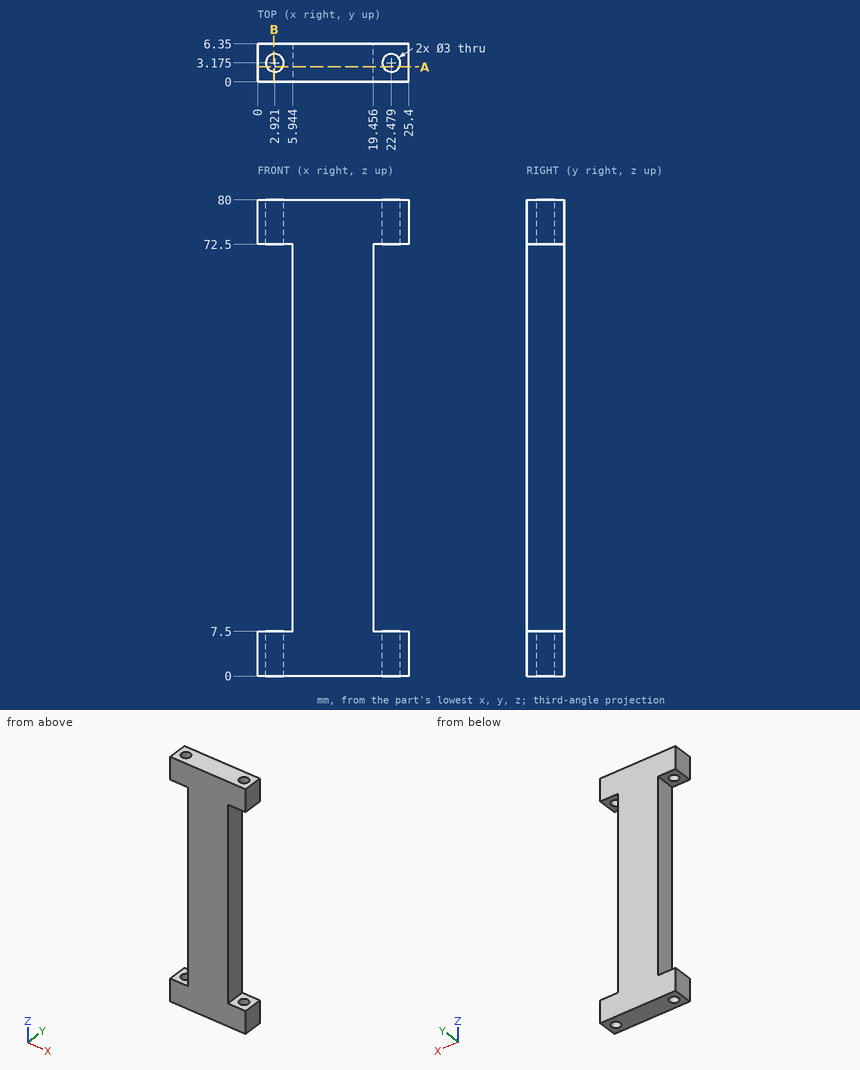
Here's the drawing with two shaded views (mm, measured from the low corner). I have some questions. Coordinates: 2 decimals unless noted, no trailing zeros. Loops run counter-clockwise (first coordinate to the right, second up) from the corner with the lowest first, then second, coordinate; pieces in that order, holes last. Notation, with made-up numbers: (65, 69) -> (79, 69) arc R18 ccw to (79, 86) -> close; hole circle Ø10 at (45.5, -36). An arc over 180 degrees is marked (long way). Answer in a Markdown table with one row per item.
(1) Imagine slicing it at A-A (y = 2.5). List the corners of the cut face in (x, z) for me, plus the area to 3 significant figures.
Results found:
| item | result |
|---|---|
| outline | (0, 0) -> (1.58, 0) -> (1.58, 7.5) -> (0, 7.5) -> close; (0, 72.5) -> (1.58, 72.5) -> (1.58, 80) -> (0, 80) -> close; (4.26, 0) -> (21.14, 0) -> (21.14, 7.5) -> (19.46, 7.5) -> (19.46, 72.5) -> (21.14, 72.5) -> (21.14, 80) -> (4.26, 80) -> (4.26, 72.5) -> (5.94, 72.5) -> (5.94, 7.5) -> (4.26, 7.5) -> close; (23.82, 0) -> (25.4, 0) -> (25.4, 7.5) -> (23.82, 7.5) -> close; (23.82, 72.5) -> (25.4, 72.5) -> (25.4, 80) -> (23.82, 80) -> close |
| area | 1,180 mm^2 |
(2) Imagine slicing it at B-B (x = 2.75). Give the number of separate pieces and of enclosed holes in the cut face.
Results found:
| item | result |
|---|---|
| separate pieces | 4 |
| enclosed holes | 0 |
(3) Will these pins go through, and if not, where does the flat tip stop? pin 1 Ø1 at (y, z) = (2.5, 24) entering from -X; pin 2 Ø1.9 at (y, z) = (4.5, 33) entering from +X.
Results found:
| item | result |
|---|---|
| pin 1 | stops at x = 5.94 |
| pin 2 | stops at x = 19.46 |
(4) If I drill on probe 1 along Z at (x, y) = (23.5, 1.5); probe 2 along X at (y, z) = (1, 11), over which ranges is the centre line in solid material (lowest first)?
Results found:
| item | result |
|---|---|
| probe 1 | z = 0 to 7.5, 72.5 to 80 |
| probe 2 | x = 5.94 to 19.46 |
